```python
from build123d import *

# Parameters (mm, degrees)
F0_W          = 78.1559385359
F0_H          = 43.0713370442
F1_DEPTH      = 38.1
F2_R          = 18.2210344627
F3_DEPTH      = 55.88
F3_DEPTH_BACK = 12.7
F5_DEPTH      = 68.581
F7_DEPTH      = 68.581
F8_R          = 4.084024571
F8_R_2        = 4.0339119635
F9_DEPTH      = 38.101


with BuildPart() as f1:
    # F0 (on Top) → F1 (new body)
    with BuildSketch(Plane.XY):
        with Locations((2.2819247097, -1.4262031764)):
            Rectangle(F0_W, F0_H)
    extrude(amount=F1_DEPTH)

    # F2 (on face) → F3 (join, two sides)
    with BuildSketch(Plane.XZ.offset(22.9618716985)) as f3_sk:
        with Locations((2.2819247097, 38.1)):
            Circle(F2_R)
    extrude(amount=-F3_DEPTH)
    extrude(f3_sk.sketch, amount=F3_DEPTH_BACK)

    # F4 (on face) → F5 (cut, through all)
    with BuildSketch(Plane(origin=(0, 32.9181283015, 0), x_dir=(-1, 0, 0), z_dir=(0, 1, 0))):
        with BuildLine():
            ThreePointArc((-10.0195623191, 48.5884337417), (-8.1567843282, 26.4653834359), (10.7518114442, 38.1))
            ThreePointArc((10.7518114442, 38.1), (9.3526918544, 43.9748596185), (5.4557128998, 48.5884337417))
            Line((5.4557128998, 48.5884337417), (-10.0195623191, 48.5884337417))
        make_face()
        with BuildLine():
            Line((-10.0195623191, 48.5884337417), (5.4557128998, 48.5884337417))
            ThreePointArc((5.4557128998, 48.5884337417), (-2.2819247097, 51.1337361539), (-10.0195623191, 48.5884337417))
        make_face()
        with BuildLine():
            ThreePointArc((-10.0195623191, 48.5884337417), (-2.2819247097, 51.1337361539), (5.4557128998, 48.5884337417))
            Line((5.4557128998, 48.5884337417), (12.6177012767, 48.5884337417))
            ThreePointArc((12.6177012767, 48.5884337417), (-2.2819247097, 77.2969690713), (-17.1815506961, 48.5884337417))
            Line((-17.1815506961, 48.5884337417), (-10.0195623191, 48.5884337417))
        make_face()
    extrude(amount=-F5_DEPTH, mode=Mode.SUBTRACT)

    # F6 (on face) → F7 (cut, through all)
    with BuildSketch(Plane(origin=(0, 32.9181283015, 0), x_dir=(-1, 0, 0), z_dir=(0, 1, 0))):
        with BuildLine():
            ThreePointArc((15.9390762318, 38.0650488792), (-2.2819247097, 57.0049656909), (-20.5029256512, 38.0650488792))
            Line((-20.5029256512, 38.0650488792), (15.9390762318, 38.0650488792))
        make_face()
    extrude(amount=-F7_DEPTH, mode=Mode.SUBTRACT)

    # F8 (on face) → F9 (cut, through all)
    with BuildSketch(Plane.XY.offset(38.1)):
        with Locations((35.0845977664, 0)):
            Circle(F8_R)
        with Locations((-30.8059900999, 0)):
            Circle(F8_R_2)
    extrude(amount=-F9_DEPTH, mode=Mode.SUBTRACT)


solid = f1.part
```
Geometry: final body of the model. Coordinates: model frame, mm. A direction names the side the tool comes from. Coordinates: 2 decimals unless noted, no trailing zeros. Write each loop counter-clockwise with the first axis right and the second up, starting at its lowest first coordinate (ties: lowest second). Pieces come first, ordered by that corner, then holes. Notation, with made-up numbers: M 80,12.5 L 134,12.5 A24 cw 134,44.5 Z; hole C -4.75,-5.75 d8. An arc over 180 degrees is marked long. Use CSV: the item, a comma, the result in double quotes. Start each with the question number.
1. Mould query, pull axis X, two halves, no side actions, for faces 1 (the face through (30.8, -1.1, 38.1)), 2 (the face through (2.57, -0.89, 25.07)), 3 (the face through (1.882, 26.603, 19.883)). Classes: pulls with the +X half, pulls with the -X half, needs draft (parallel to the pull), parting line crosses it, or undercut.
2. First-contact query: P1, Ø6, axis at x = -11, z = 4.5, coming from the -Y side; P2, Ø6, axis at x = 18.5, z = 13, coming from the +Y side; P3, Ø1.6, axis at x = -13, y = 4, coming from the +Z side. Flat tips, straight axial feed; report the tip coordinate or a pass-through.
3. Reachability of faces 4 (the face through (2, -22.962, 15)), 5 (the face through (2, 20.109, 15)), 6 (the face through (-26.5, -1.1, 38.1)) from +Z, -Z, +X, -X, +Y, -Y: full face, straight path, thin tool, end or side. Return the list, or none.
4. Cut plane B-B on z = 32. Return the cut outline in (x, y).
5. Cut plane D-D on x = 25.5. Return the cut outline in (y, z), plus the area to 3 significant figures.
6. Cut plane A-A on y = 0. Count the separate pieces of the cut face and the enclosed holes in it, plus the area to 3 significant figures.
7. Ray query, probe 1 along Y at (x, z) = (34.5, 28.5); probe 2 along Y at (x, z) = (-6, 9); probe 3 along Z at (x, y) = (17, 14.5). Return the intervals inside material, ascending.
Entries:
1,face 1,"needs draft"
1,face 2,"undercut"
1,face 3,"parting line crosses it"
2,P1,"y = -22.96"
2,P2,"y = 20.11"
2,P3,"z = 38.07"
3,face 4,"-Z, -Y"
3,face 5,"-Z, +Y"
3,face 6,"+Z, +X, -X, +Y, -Y"
4,outline,"M -36.8,-22.96 L -14.89,-22.96 L -14.89,-35.66 L -9.24,-35.66 L -9.24,32.92 L -14.89,32.92 L -14.89,20.11 L -36.8,20.11 Z; M 13.8,-35.66 L 19.45,-35.66 L 19.45,-22.96 L 41.36,-22.96 L 41.36,20.11 L 19.45,20.11 L 19.45,32.92 L 13.8,32.92 Z; hole C -30.81,0 d8.07; hole C 35.08,0 d8.17"
5,outline,"M -22.96,0 L 20.11,0 L 20.11,38.1 L -22.96,38.1 Z"
5,area,"1,640 mm²"
6,separate pieces,"3"
6,enclosed holes,"0"
6,area,"2,090 mm²"
7,probe 1,"-22.96 to -4.04, 4.04 to 20.11"
7,probe 2,"-22.96 to 20.11"
7,probe 3,"0 to 38.07"
